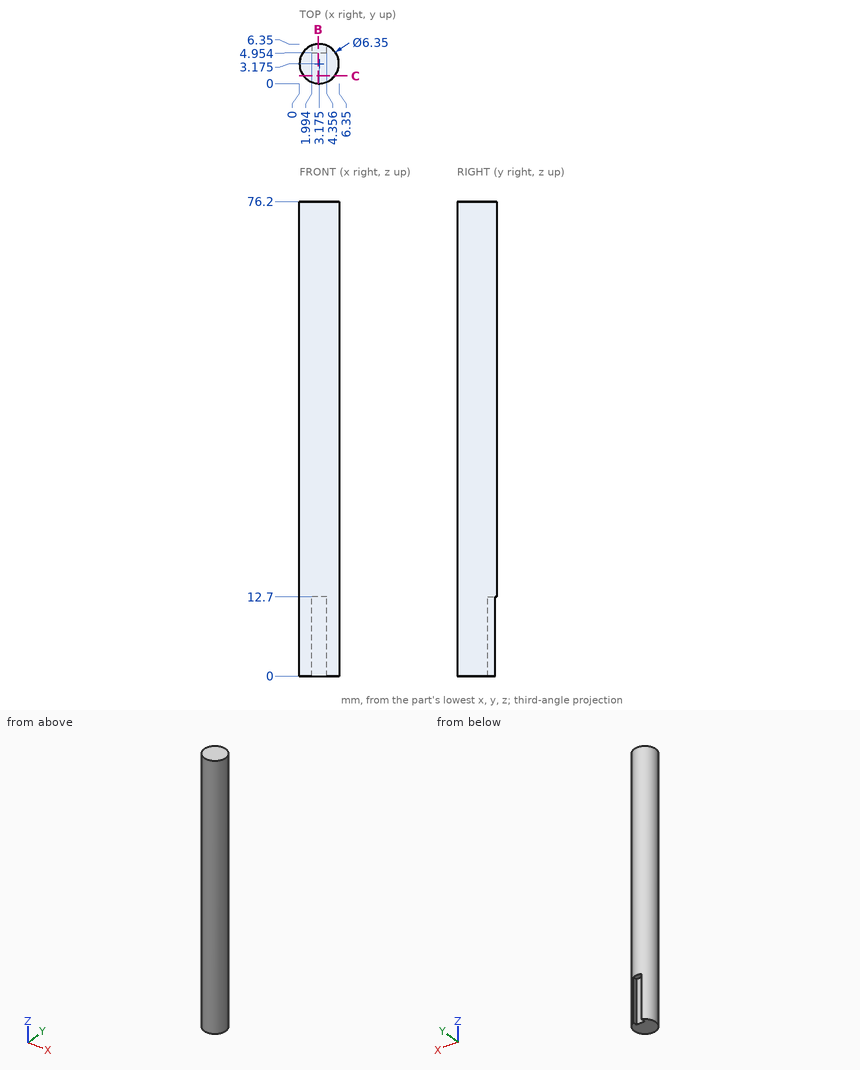
Check sheet for the drawn part. Datum: minimum x, y, z corner. Units: mm. Coordinates: 2 decimals unless noted, no trailing zeros. Loops run counter-clockwise (first coordinate to the right, second up) from the corner with the lowest first, then second, coordinate; pieces in that order, holes last. Notation, with made-up numbers: (38, -24) - (45, -24) arc R32 ccw to (45, 14) - close; hole circle Ø3 at (61.25, 72.25). An arc over 180 degrees is marked (long way). Put each result on its own line as item: value.
Item 1: Section check B-B (x = 3). Enter the section's corners in (y, z) (1 decimal).
Conclusion:
outline: (0, 0) - (5, 0) - (5, 12.7) - (6.3, 12.7) - (6.3, 76.2) - (0, 76.2) - close
Item 2: Scan lines: line 1 along Y through (x, z) = (3, 59) (1 decimal); line 2 along Z through (x, y) = (2.25, 5). Record each from-to range of solid material in increasing order.
Conclusion:
line 1: y = 0 to 6.3
line 2: z = 12.7 to 76.2
Item 3: Section check C-C (y = 1.25). Enter the section's corners in (x, z).
Conclusion:
outline: (0.65, 0) - (5.7, 0) - (5.7, 76.2) - (0.65, 76.2) - close
Item 4: Gauge pin test, flat ends, axial feed: pin 1 Ø1.3 at (y, z) = (5.5, 6.5) entering from +X; pin 2 Ø0.9 at (y, z) = (5.5, 5.5) entering from -X; pin 3 Ø1.9 at (x, z) = (2.5, 7) entering from +Y. Record the tip position at first contact, or that the pin passes through.
Conclusion:
pin 1: stops at x = 5.87
pin 2: stops at x = 0.61
pin 3: stops at y = 6.12
